Design review of the part built by this model. Coordinates are the model's own, in mm. A direction names the side the tool comes from. Coordinates: 2 decimals unless noted, no trailing zeros. Loops run counter-clockwise (first coordinate to the right, second up) from the corner with the lowest first, then second, coordinate; pieces in that order, holes last. Notation, with made-up numbers: (36.25, 16.25) -> (47.25, 16.25) arc R18 ccw to (47.25, 39.25) -> close; hole circle Ø4 at (-39.5, 25). An arc over 180 degrees is marked (long way). Answer in a Markdown table with one row per item.
Autodesk Inventor part; units mm, degrees
ref_plane "YZ Plane" through (0, 0, 0) normal (1, 0, 0) x (0, 1, 0)
ref_plane "XZ Plane" through (0, 0, 0) normal (0, 1, 0) x (-1, 0, 0)
ref_plane "XY Plane" through (0, 0, 0) normal (0, 0, 1) x (1, 0, 0)
sketch "Sketch1" plane through (0, 0, 0) normal (0, 1, 0) x (-1, 0, 0)
  line L0 (0, 0) -> (20, 0)
  line L1 (20, 0) -> (20, -3)
  line L2 (20, -3) -> (0, -3)
  line L3 (0, -3) -> (0, 0)
  line L4 (0, 0) -> (3, 0)
  line L5 (3, 0) -> (3, -20)
  line L6 (3, -20) -> (0, -20)
  line L7 (0, -20) -> (0, 0)
  dimension "d0" = 3
  dimension "d1" = 3
  dimension "d2" = 20
  dimension "d3" = 20
extrude "Extrusion1" add sketch "Sketch1" along normal blind 50
fillet "Fillet1" radius 2 1 edges at (-3, 25, -3)
fillet "Fillet2" radius 5 1 edges at (0, 25, 0)
sketch "Sketch2" plane through (-3, 0, -20) normal (-1, 0, 0) x (0, 0, 1)
  line L0 (0, 50) -> (15, 50)
  line L1 (0, 0) -> (15, 0)
  line L2 (0, 0) -> (0, 50)
  point P0 (20, 0)
  point P1 (7.5, 42.5)
  point P2 (7.5, 7.5)
  dimension "d8" = 7.5
  dimension "d9" = 7.5
  dimension "d10" = 35
  dimension "d11" = 7.5
hole "Hole1" at (-3, 42.5, -12.5) at (-3, 7.5, -12.5) direction (1, 0, 0) diameter 4.5 end through all
sketch "Sketch3" plane through (-20, 0, -3) normal (0, 0, -1) x (-1, 0, 0)
  line L0 (-15, 50) -> (0, 50)
  line L1 (-15, 0) -> (0, 0)
  line L2 (0, 0) -> (0, 50)
  point P0 (-20, 0)
  point P1 (-7.5, 42.5)
  point P2 (-7.5, 7.5)
  dimension "d19" = 7.5
  dimension "d20" = 7.5
  dimension "d21" = 7.5
hole "Hole2" at (-12.5, 42.5, -3) at (-12.5, 7.5, -3) direction (0, 0, 1) diameter 4.5 end through all
equation "\"d1\" = d0"
equation "\"d3\" = d2"
properties part number "Pancake_Angle Bracket" material "Aluminum 6061"
(1) Take a section at C-C on x = -12.5. Give the boundary of the cut face in (y, z).
Evaluation:
| item | result |
|---|---|
| outline | (0, -3) -> (5.25, -3) -> (5.25, 0) -> (0, 0) -> close; (9.75, -3) -> (40.25, -3) -> (40.25, 0) -> (9.75, 0) -> close; (44.75, -3) -> (50, -3) -> (50, 0) -> (44.75, 0) -> close |
(2) Take a section at D-D on y = 30. Give the boundary of the cut face in (x, z), and give its area (3 significant figures).
Evaluation:
| item | result |
|---|---|
| outline | (-20, -3) -> (-5, -3) arc R2 cw to (-3, -5) -> (-3, -20) -> (0, -20) -> (0, -5) arc R5 ccw to (-5, 0) -> (-20, 0) -> close |
| area | 106 mm² |
(3) Take a section at A-A on z = -12.5. Give the boundary of the cut face in (x, y).
Evaluation:
| item | result |
|---|---|
| outline | (-3, 0) -> (0, 0) -> (0, 5.25) -> (-3, 5.25) -> close; (-3, 9.75) -> (0, 9.75) -> (0, 40.25) -> (-3, 40.25) -> close; (-3, 44.75) -> (0, 44.75) -> (0, 50) -> (-3, 50) -> close |
(4) To check wall thickness, follow probe 1 along Y at (x, z) = (-12.5, -2.15); probe 2 along Y at (x, z) = (-13.75, -2.25); probe 3 along X at (y, z) = (13, -10.25). State the ranges of each line that lie inside material, in increasing order.
Evaluation:
| item | result |
|---|---|
| probe 1 | y = 0 to 5.25, 9.75 to 40.25, 44.75 to 50 |
| probe 2 | y = 0 to 5.63, 9.37 to 40.63, 44.37 to 50 |
| probe 3 | x = -3 to 0 |
(5) Draft analysis for pull direction X (two halves, no side actions). For faces 1 (the flat face through (0, 25, -13)), 2 (the flat face through (-13, 25, -3)), 3 (the cylindrical face through (-14.73, 7.21, -1.48)), state which applies: pulls with the +X half, pulls with the -X half, needs draft (parallel to the pull), parting line crosses it, or undercut.
Evaluation:
| item | result |
|---|---|
| face 1 | pulls with the +X half |
| face 2 | needs draft |
| face 3 | undercut |
(6) Tool access review of faces 4 (the cylindrical face through (-2, 25, -1)), 5 (the flat face through (-3, 25, -12)): name each direction out of +Z, -Z, +X, -X, +Y, -Y from which nothing blocks a thin tool from reaching the whole face with its end or side.
Evaluation:
| item | result |
|---|---|
| face 4 | +Z, +X, +Y, -Y |
| face 5 | -Z, -X, +Y, -Y |
(7) For pin 1 (1 mm diameter, centred on y = 25, z = -13, fed in from -X); pin 2 (12 mm diameter, centred on x = -14, y = 24, fed in from -Z); pin 3 (6 mm diameter, centred on x = -17.5, z = -7, fed in from +Y), all flat-tipped, find the tip position at first contact; note any pin that passes through.
Evaluation:
| item | result |
|---|---|
| pin 1 | stops at x = -3 |
| pin 2 | stops at z = -3 |
| pin 3 | passes through |
(8) Take a section at B-B on y = 42.5. Give the boundary of the cut face in (x, z), and give its area (3 significant figures).
Evaluation:
| item | result |
|---|---|
| outline | (-20, -3) -> (-14.75, -3) -> (-14.75, 0) -> (-20, 0) -> close; (-10.25, -3) -> (-5, -3) arc R2 cw to (-3, -5) -> (-3, -10.25) -> (0, -10.25) -> (0, -5) arc R5 ccw to (-5, 0) -> (-10.25, 0) -> close; (-3, -20) -> (0, -20) -> (0, -14.75) -> (-3, -14.75) -> close |
| area | 79.5 mm² |
